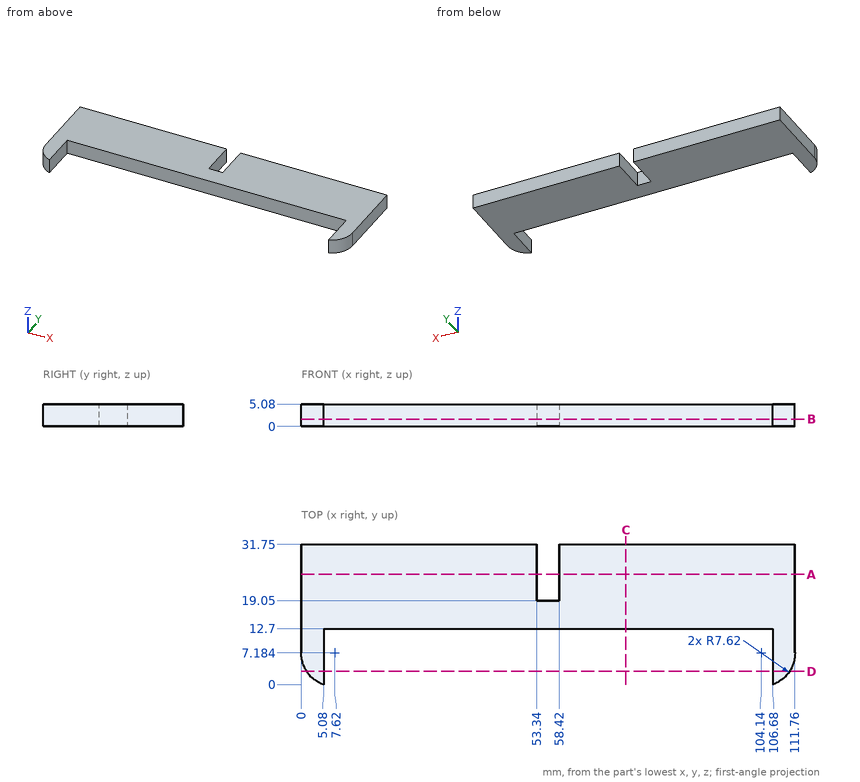
Verification items for this drawing (mm, ordinates from the low corner). Give positions to 0.01 mm unless a question says otherwise; leave off trailing zeros. Write each loop counter-clockwise with the first axis right and the second up, starting at its lowest first coordinate (ties: lowest second). Pieces come first, ordered by that corner, then holes. Notation, with made-up numbers: (76, -35.5) -> (119, -35.5) arc R16 cw to (119, -12.5) -> close; hole circle Ø6 at (1.25, 12). An arc over 180 degrees is marked (long way). Use CSV: the item, a comma, the result in double quotes.
(1) Sectioned sample at A-A (y = 25). Record the cut outline in (x, z).
Derived:
outline,"(0, 0) -> (53.34, 0) -> (53.34, 5.08) -> (0, 5.08) -> close; (58.42, 0) -> (111.76, 0) -> (111.76, 5.08) -> (58.42, 5.08) -> close"
(2) Go/stop test with flat-tipped pins: pin 1 (3 mm diameter, centred on x = 18.5, z = 3.5, fed in from -Y); pin 2 (1.5 mm diameter, centred on x = 55, z = 3.5, fed in from +Y); pin 3 (2.5 mm diameter, centred on y = 5.5, z = 3, fed in from +X). Record where each tip stops, or that it passes through.
Derived:
pin 1,"stops at y = 12.7"
pin 2,"stops at y = 19.05"
pin 3,"stops at x = 111.75"
(3) Sectioned sample at D-D (y = 3). Record the cut outline in (x, z).
Derived:
outline,"(1.25, 0) -> (5.08, 0) -> (5.08, 5.08) -> (1.25, 5.08) -> close; (106.68, 0) -> (110.51, 0) -> (110.51, 5.08) -> (106.68, 5.08) -> close"
(4) Material ranges on L1, parallel to X at y = 29, z = 3.2; L2, parallel to X at y = 10.5, z = 4.55; L3, parallel to Y at x = 59, z = 4.55, recorded low to high.
Derived:
L1,"x = 0 to 53.34, 58.42 to 111.76"
L2,"x = 0 to 5.08, 106.68 to 111.76"
L3,"y = 12.7 to 31.75"
(5) Sectioned sample at B-B (z = 1.65). Record the cut outline in (x, y).
Derived:
outline,"(0, 7.18) arc R7.62 ccw to (5.08, 0) -> (5.08, 12.7) -> (106.68, 12.7) -> (106.68, 0) arc R7.62 ccw to (111.76, 7.18) -> (111.76, 31.75) -> (58.42, 31.75) -> (58.42, 19.05) -> (53.34, 19.05) -> (53.34, 31.75) -> (0, 31.75) -> close"
(6) Sectioned sample at C-C (x = 73.5). Record the cut outline in (y, z), plus the area to 3 significant figures.
Derived:
outline,"(12.7, 0) -> (31.75, 0) -> (31.75, 5.08) -> (12.7, 5.08) -> close"
area,"96.8 mm^2"
